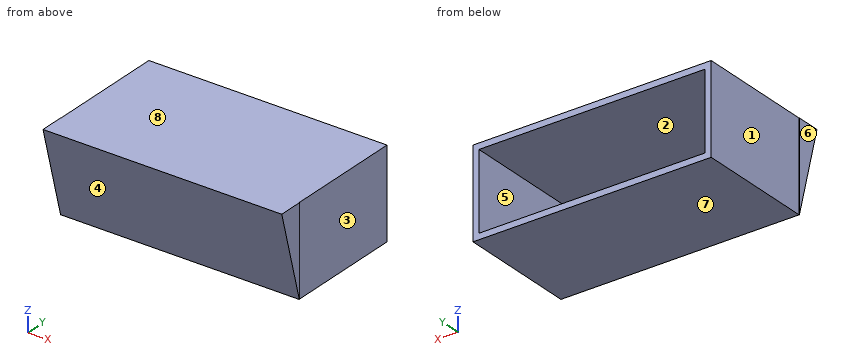
```python
from build123d import *

# Parameters (mm, degrees)
F0_W        = 79.8
F0_H        = 29.8
F1_DEPTH    = 20
F3_DEPTH    = 40
F4_T        = 2
F4_T3_DEPTH = 33.8


# Not quite as in the source:
# - a shell that OpenCascade refuses in one call is made with other operations: the cavity is built on its own and cut out


with BuildPart() as f1:
    # F0 (on Front) → F1 (new body, symmetric)
    with BuildSketch(Plane.XZ):
        Rectangle(F0_W, F0_H)
    extrude(amount=F1_DEPTH, both=True)

    # F2 (on Right) → F3 (join, symmetric)
    with BuildSketch(Plane.YZ):
        Polygon((-28, 14.9), (-20, -14.9), (-20, 14.9), align=None)
    extrude(amount=F3_DEPTH, both=True)

    # F4: shell of thickness 2, made by hand


with BuildPart() as f4_core1:
    # F4_t2: copy of F1
    add(f1.part)

    # the walls: a layer under each face that stays
    f4_faces = [f4_core1.faces().sort_by_distance(p)[0] for p in [
        (0, -24, 0),
        (-40, -24, 9.9333333333),
        (-39.95, -20, 0),
        (0, 0, -14.9),
        (39.95, -20, 0),
        (40, -24, 9.9333333333),
        (0, -4, 14.9),
        (-39.9, 0, 0),
        (39.9, 0, 0),
    ]]
    thicken(f4_faces, amount=-F4_T, mode=Mode.SUBTRACT)

    # F4_s4 → F4_t3 (cut)
    with BuildSketch(Plane.XY.offset(-16.9)):
        Polygon((-39.92, -19.98), (-39.9, -22), (-37.9, -22), (-37.9, -20), align=None)
        Polygon((39.92, -19.98), (39.9, -22), (37.9, -22), (37.9, -20), align=None)
    extrude(amount=F4_T3_DEPTH, mode=Mode.SUBTRACT)


with BuildPart() as f1_1:
    add(f1.part)

    # what is left inside the walls is the cavity
    f4_cavity = [f4_core1.part.solids().sort_by_distance(p)[0] for p in [
        (-12.666667, -2.696136, 12.88),
    ]]
    add(f4_cavity, mode=Mode.SUBTRACT)


solid = f1_1.part
```
Geometry check sheet. Reference: the model listing, model coordinates, mm. Face numbers are marked on the shaded views. A direction names the side the tool comes from. Round coordinates to 2 decimals unless told otherwise and drop trailing zeros. Loops run counter-clockwise (first coordinate to the right, second up) from the corner with the lowest first, then second, coordinate; pieces in that order, holes last. Notation, with made-up numbers: (71.25, 66) - (90.25, 66) arc R23 ccw to (90.25, 74) - close; hole circle Ø7 at (83.25, 5). An arc over 180 degrees is marked (long way). Use a Markdown table: item, result.
Q1. Cross-section at D-D on y = -24. Record the cut outline in (x, z), plus the area to 3 significant figures.
Solutions:
| item | result |
|---|---|
| outline | (-40, 0) - (40, 0) - (40, 14.9) - (-40, 14.9) - close; hole (-38, 7.71) - (38, 7.71) - (38, 12.9) - (-38, 12.9) - close |
| area | 798 mm2 |
Q2. Material ranges on line 1 (Z direction, x = 35, y = -7); line 2 (X direction, y = -6.5, z = -10); line 3 (X direction, y = -21.5, z = 7.5), recorded low to high.
Solutions:
| item | result |
|---|---|
| line 1 | z = -14.9 to -12.9, 12.9 to 14.9 |
| line 2 | x = -39.9 to -37.9, 37.9 to 39.9 |
| line 3 | x = -40 to -37.9, 37.9 to 40 |
Q3. Go/stop test with flat-tipped pins: P1, Ø1.5, axis at x = -9, z = -4.5, coming from the -Y side; P2, Ø2, axis at y = 1, z = 6.5, coming from the -X side; P3, Ø7.5, axis at y = -9.5, z = -4.5, coming from the +X side. Record where each tip stops, or that it passes through.
Solutions:
| item | result |
|---|---|
| P1 | stops at y = -22.99 |
| P2 | stops at x = -39.9 |
| P3 | stops at x = 39.9 |
Q4. Cross-section at A-A on y = -11. Record the cut outline in (x, z), plus the area to 3 significant figures.
Solutions:
| item | result |
|---|---|
| outline | (-39.9, -14.9) - (39.9, -14.9) - (39.9, 14.9) - (-39.9, 14.9) - close; hole (-37.9, -12.9) - (37.9, -12.9) - (37.9, 12.9) - (-37.9, 12.9) - close |
| area | 422 mm2 |
Q5. Access from +Z, -Z, +X, -X, +Y, -Y to the whole of each face (thin tool, end or side, straight path). Record for the marked faces 1, 2, 3 and 4.
Solutions:
| item | result |
|---|---|
| face 1 | +Z, -Z, -X, +Y |
| face 2 | +Y |
| face 3 | +Z, -Z, +X, +Y |
| face 4 | -Z, +X, -X, -Y |
Q6. Cross-section at C-C on z = 6.5. Record the cut outline in (x, y), plus the area to 3 significant figures.
Solutions:
| item | result |
|---|---|
| outline | (-40, -25.74) - (40, -25.74) - (40, -20) - (39.9, -20) - (39.9, 20) - (37.9, 20) - (37.9, -22) - (38, -22) - (38, -23.67) - (-38, -23.67) - (-38, -22) - (-37.9, -22) - (-37.9, 20) - (-39.9, 20) - (-39.9, -20) - (-40, -20) - close |
| area | 341 mm2 |
Q7. Draft check along Z on the marked faces 5, 6, 7 and 8. Enter one of: released by +Z, released by -Z, zero draft, split by the parting line, or undercut.
Solutions:
| item | result |
|---|---|
| face 5 | undercut |
| face 6 | zero draft |
| face 7 | released by -Z |
| face 8 | released by +Z |
Q8. Cross-section at B-B on x = -9. Record the cut outline in (y, z), plus the area to 3 significant figures.
Solutions:
| item | result |
|---|---|
| outline | (-28, 14.9) - (-20, -14.9) - (20, -14.9) - (20, -12.9) - (-18.47, -12.9) - (-25.39, 12.9) - (20, 12.9) - (20, 14.9) - close |
| area | 229 mm2 |
